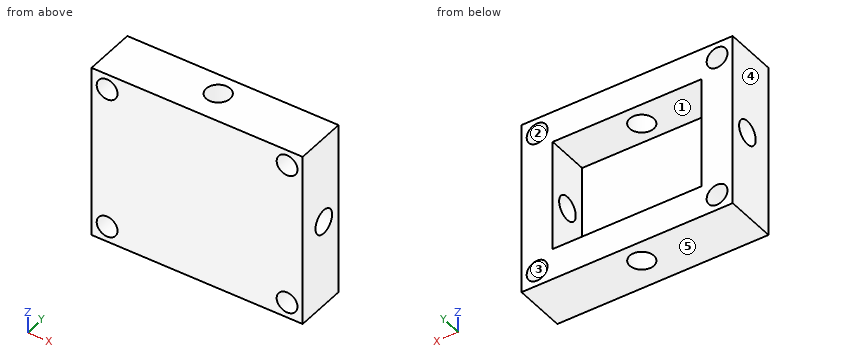
from build123d import *

# Parameters (mm, degrees)
SKETCH1_W               = 36.068
SKETCH1_H               = 29.718
SKETCH1_W_2             = 25.4
SKETCH1_H_2             = 19.05
BOSS_EXTRUDE3_DEPTH     = 7.2898
SKETCH4_W               = 36.068
SKETCH4_H               = 29.718
BOSS_EXTRUDE4_DEPTH     = 1.5875
SKETCH5_R               = 1.778
CUT_EXTRUDE2_DEPTH      = 9.525
CUT_EXTRUDE3_DEPTH      = 40.684149091
CUT_EXTRUDE3_DEPTH_BACK = 40.684149091
SKETCH6_R               = 2.0574
SKETCH7_R               = 2.0574
CUT_EXTRUDE4_DEPTH      = 36.51796537


with BuildPart() as part:
    # Sketch1 → Boss-Extrude3 (new body)
    with BuildSketch(Plane(origin=(0, 0, 0), x_dir=(1, 0, 0), z_dir=(0, 1, 0))):
        Rectangle(SKETCH1_W, SKETCH1_H)
        Rectangle(SKETCH1_W_2, SKETCH1_H_2, mode=Mode.SUBTRACT)
    extrude(amount=BOSS_EXTRUDE3_DEPTH)

    # Sketch4 → Boss-Extrude4 (add)
    with BuildSketch(Plane.XZ):
        Rectangle(SKETCH4_W, SKETCH4_H)
    extrude(amount=BOSS_EXTRUDE4_DEPTH)

    # Sketch5 → Cut-Extrude2 (cut)
    with BuildSketch(Plane(origin=(0, 7.2898, 0), x_dir=(1, 0, 0), z_dir=(0, 1, 0))):
        with Locations(Location((-15.367, 12.192, 0), (0, 0, 270))):
            Circle(SKETCH5_R)
        with Locations(Location((15.367, 12.192, 0), (0, 0, 270))):
            Circle(SKETCH5_R)
        with Locations(Location((15.367, -12.192, 0), (0, 0, 270))):
            Circle(SKETCH5_R)
        with Locations(Location((-15.367, -12.192, 0), (0, 0, 270))):
            Circle(SKETCH5_R)
    extrude(amount=-CUT_EXTRUDE2_DEPTH, mode=Mode.SUBTRACT)

    # Sketch6 → Cut-Extrude3 (cut, two sides: drawn at the far end of the back side and taken through both)
    with BuildSketch(Plane(origin=(18.034, 0, 0), x_dir=(0, 0, -1), z_dir=(1, 0, 0)).offset(-CUT_EXTRUDE3_DEPTH_BACK)):
        with Locations((0, 3.6449)):
            Circle(SKETCH6_R)
    extrude(amount=CUT_EXTRUDE3_DEPTH + CUT_EXTRUDE3_DEPTH_BACK, mode=Mode.SUBTRACT)

    # Sketch7 → Cut-Extrude4 (cut, through all)
    with BuildSketch(Plane.XY.offset(14.859)):
        with Locations((0, 3.6449)):
            Circle(SKETCH7_R)
    extrude(amount=-CUT_EXTRUDE4_DEPTH, mode=Mode.SUBTRACT)


solid = part.part
Check sheet for the modelled part. Datum: model origin and axes. Units: mm. Face numbers are marked on the shaded views. A direction names the side the tool comes from. Round coordinates to 2 decimals unless told otherwise and drop trailing zeros. Write each loop counter-clockwise with the first axis right and the second up, starting at its lowest first coordinate (ties: lowest second). Pieces come first, ordered by that corner, then holes. Notation, with made-up numbers: (44, 21) -> (56, 21) arc R12 cw to (56, 43) -> close; hole circle Ø10 at (29, 88.5). An arc over 180 degrees is marked (long way). Answer as CSV lines item,"result". Start each with the question number.
1) Section check B-B on z = 0. Enter the section's corners in (x, y), and give its area (3 significant figures).
2) Section check C-C on y = 5.25. Enter the section's corners in (x, z) (3 decimals), and give its area (3 significant figures).
3) Tool access check on the marked faces 1 and 2. Record the directions out of +Z, -Z, +X, -X, +Y, -Y that give a thin tool (end or side, any length) a straight path to the whole face; none if there is none.
4) Release check for a two-part mould opening along X. For the marked faces 3, 4 and 5 record: pulls with the +X half, pulls with the -X half, needs draft (parallel to the pull), parting line crosses it, or undercut.
5) Section check D-D on x = -14. Enter the section's corners in (y, z), and give its area (3 significant figures).
6) Go/stop test with a flat-tipped pin: P1, Ø9.5, axis at x = 4.5, z = 2.5, coming from the +Y side. Record where the tip stops, or that it passes through.
7) Section check A-A on x = 0. Enter the section's corners in (y, z) (1 decimal), and give its area (3 significant figures).
8) Material ranges on line 1 (X direction, y = 6.75, z = 12.25); line 2 (X direction, y = 2.5, z = 3); line 3 (Z direction, x = -8, y = 2.25) (3 decimals), recorded low to high. Write a range as from..to.
Found:
1,outline,"(-18.03, -1.59) -> (18.03, -1.59) -> (18.03, 1.59) -> (12.7, 1.59) -> (12.7, 0) -> (-12.7, 0) -> (-12.7, 1.59) -> (-18.03, 1.59) -> close; (-18.03, 5.7) -> (-12.7, 5.7) -> (-12.7, 7.29) -> (-18.03, 7.29) -> close; (12.7, 5.7) -> (18.03, 5.7) -> (18.03, 7.29) -> (12.7, 7.29) -> close"
1,area,"91.1 mm^2"
2,outline,"(-18.034, -14.859) -> (-1.287, -14.859) -> (-1.287, -9.525) -> (-12.7, -9.525) -> (-12.7, -1.287) -> (-18.034, -1.287) -> close; (-18.034, 1.287) -> (-12.7, 1.287) -> (-12.7, 9.525) -> (-1.287, 9.525) -> (-1.287, 14.859) -> (-18.034, 14.859) -> close; (1.287, -14.859) -> (18.034, -14.859) -> (18.034, -1.287) -> (12.7, -1.287) -> (12.7, -9.525) -> (1.287, -9.525) -> close; (1.287, 9.525) -> (12.7, 9.525) -> (12.7, 1.287) -> (18.034, 1.287) -> (18.034, 14.859) -> (1.287, 14.859) -> close; hole circle Ø3.556 at (-15.367, -12.192); hole circle Ø3.556 at (-15.367, 12.192); hole circle Ø3.556 at (15.367, -12.192); hole circle Ø3.556 at (15.367, 12.192)"
2,area,"493 mm^2"
3,face 1,"+Y"
3,face 2,"+Y, -Y"
4,face 3,"undercut"
4,face 4,"pulls with the -X half"
4,face 5,"needs draft"
5,outline,"(-1.59, -14.86) -> (7.29, -14.86) -> (7.29, -13.33) -> (-1.59, -13.33) -> close; (-1.59, -11.06) -> (7.29, -11.06) -> (7.29, 11.06) -> (-1.59, 11.06) -> close; (-1.59, 13.33) -> (7.29, 13.33) -> (7.29, 14.86) -> (-1.59, 14.86) -> close; hole circle Ø4.11 at (3.64, 0)"
5,area,"210 mm^2"
6,P1,"stops at y = 0"
7,outline,"(-1.6, -14.9) -> (1.6, -14.9) -> (1.6, -9.5) -> (0, -9.5) -> (0, 9.5) -> (1.6, 9.5) -> (1.6, 14.9) -> (-1.6, 14.9) -> close; (5.7, -14.9) -> (7.3, -14.9) -> (7.3, -9.5) -> (5.7, -9.5) -> close; (5.7, 9.5) -> (7.3, 9.5) -> (7.3, 14.9) -> (5.7, 14.9) -> close"
7,area,"81.0 mm^2"
8,line 1,"x = -18.03..-17.14, -13.59..13.59, 17.14..18.03"
8,line 2,"x = -18.03..-12.7, 12.7..18.03"
8,line 3,"z = -14.859..-9.525, 9.525..14.859"
